```python
from build123d import *

# Parameters (mm, degrees)
F0_W     = 24
F0_H     = 16
F1_DEPTH = 2
F2_W     = 1.5
F2_H     = 16
F2_H_2   = 10
F3_DEPTH = 8
F4_DEPTH = 2
F5_SIZE  = 8
F6_R     = 1


with BuildPart() as f1:
    # F0 (on Front) → F1 (new body)
    with BuildSketch(Plane.XZ):
        Rectangle(F0_W, F0_H)
    extrude(amount=F1_DEPTH)

    # F2 (on face) → F3 (join)
    with BuildSketch(Plane.XZ.offset(2)):
        Rectangle(F2_W, F2_H)
        with Locations((0, -13)):
            Rectangle(F2_W, F2_H_2)
    extrude(amount=F3_DEPTH)

    # F4 (cut): a face of the model
    f4_faces = [f1.faces().sort_by_distance(p)[0] for p in [
        (0, -2, -13),
    ]]
    extrude(f4_faces, amount=-F4_DEPTH, mode=Mode.SUBTRACT)

    # F5
    f5_edges = [f1.edges().sort_by_distance(p)[0] for p in [
        (0, -10, 8),
    ]]
    chamfer(f5_edges, length=F5_SIZE)

    # F6
    f6_edges = [f1.edges().sort_by_distance(p)[0] for p in [
        (-0.75, -2, 0),
        (0.75, -2, 0),
    ]]
    fillet(f6_edges, radius=F6_R)


solid = f1.part
```
Model file for the job. Use its own axes, mm. A direction names the side the tool comes from. Coordinates: 2 decimals unless noted, no trailing zeros. Write each loop counter-clockwise with the first axis right and the second up, starting at its lowest first coordinate (ties: lowest second). Pieces come first, ordered by that corner, then holes. Notation, with made-up numbers: (13.25, 33.25) - (61.25, 33.25) arc R7 ccw to (61.25, 46.25) - close; hole circle Ø2 at (35.25, -12.75). An arc over 180 degrees is marked (long way). One line per item, written item: value. Start each with the question number.
1. Tool access for faces 1 (the flat face through (0, -1, -8)), 2 (the flat face through (7, -2, 0)), 3 (the flat face through (-7, -2, 0)): list every direction of +Z, -Z, +X, -X, +Y, -Y with a clear straight run to the whole face (end or side of a thin tool).
2. Slice it at B-B (y = -7.75). Write the cut outline in (x, z), plus the area to 3 significant figures.
3. Flat gauge pins, fed straight in: pin 1 (3 mm diameter, centred on x = -8.5, z = -1.5, fed in from -Y); pin 2 (2 mm diameter, centred on x = 2.5, z = 4.5, fed in from +Y); pin 3 (1.6 mm diameter, centred on x = 0, z = -14, fed in from +Y); pin 4 (4 mm diameter, centred on x = -5.5, z = -11, fed in from +Y). Where does each tip first touch, or does it go through?
4. Probe line 1 (Y direction, x = 2, z = 0.75); line 2 (X direction, y = -9.5, z = -8.25). List the from-to ranges inside material, lowest first. Write a range as from..to.
5. Slice it at D-D (x = 6). Write the cut outline in (y, z), plus the area to 3 significant figures.
6. Slice it at A-A (z = 1.5). Write the cut outline in (x, y), plus the area to 3 significant figures.
7. Slice it at C-C (z = -5). Write the cut outline in (x, y).
Answers below:
1. face 1: -Z, +X, -X, +Y
1. face 2: +Z, -Z, +X, -Y
1. face 3: +Z, -Z, -X, -Y
2. outline: (-0.75, -18) - (0.75, -18) - (0.75, 2.25) - (-0.75, 2.25) - close
2. area: 30.4 mm^2
3. pin 1: stops at y = -2
3. pin 2: stops at y = 0
3. pin 3: stops at y = -4
3. pin 4: passes through
4. line 1: y = -2..0
4. line 2: x = -0.75..0.75
5. outline: (-2, -8) - (0, -8) - (0, 8) - (-2, 8) - close
5. area: 32.0 mm^2
6. outline: (-12, -2) - (-1.75, -2) arc R1 cw to (-0.75, -3) - (-0.75, -8.5) - (0.75, -8.5) - (0.75, -3) arc R1 cw to (1.75, -2) - (12, -2) - (12, 0) - (-12, 0) - close
6. area: 58.2 mm^2
7. outline: (-12, -2) - (-1.75, -2) arc R1 cw to (-0.75, -3) - (-0.75, -10) - (0.75, -10) - (0.75, -3) arc R1 cw to (1.75, -2) - (12, -2) - (12, 0) - (-12, 0) - close
